from build123d import *

# Parameters (mm, degrees)
SKETCH1_R           = 4.5
BOSS_EXTRUDE1_DEPTH = 2.4
FILLET1_R           = 3
SKETCH2_R           = 3.25
BOSS_EXTRUDE2_DEPTH = 5.5


with BuildPart() as part:
    # Sketch1 → Boss-Extrude1 (new body)
    with BuildSketch(Plane(origin=(0, 0, 0), x_dir=(1, 0, 0), z_dir=(0, 1, 0))):
        with BuildLine():
            ThreePointArc((-48.371159118, 10.670216357), (-67.382417284, 0), (-48.371159118, -10.670216357))
            Line((-48.371159118, -10.670216357), (-39.699633202, -7.41775842))
            Line((-39.699633202, -7.41775842), (-5.857739229, -16.176946436))
            ThreePointArc((-5.857739229, -16.176946436), (21.617582716, 0), (-5.857739229, 16.176946436))
            Line((-5.857739229, 16.176946436), (-39.699633202, 7.41775842))
            Line((-39.699633202, 7.41775842), (-48.371159118, 10.670216357))
        make_face()
        with BuildLine():
            Line((-11.950545902, 3), (-25.528315318, 3))
            ThreePointArc((-25.528315318, 3), (-28.882417284, 4.5), (-32.23651925, 3))
            Line((-32.23651925, 3), (-42.747756184, 3))
            Line((-42.747756184, 3), (-17.634945081, 8.68439918))
            Line((-17.634945081, 8.68439918), (-11.950545902, 3))
        make_face(mode=Mode.SUBTRACT)
        with BuildLine():
            Line((9.717339795, -8.5), (9.717339795, 8.5))
            ThreePointArc((9.717339795, 8.5), (18.217339795, 0), (9.717339795, -8.5))
        make_face(mode=Mode.SUBTRACT)
        with BuildLine():
            Line((-42.747756184, -3), (-32.23651925, -3))
            ThreePointArc((-32.23651925, -3), (-28.882417284, -4.5), (-25.528315318, -3))
            Line((-25.528315318, -3), (-11.950545902, -3))
            Line((-11.950545902, -3), (-17.634945081, -8.68439918))
            Line((-17.634945081, -8.68439918), (-42.747756184, -3))
        make_face(mode=Mode.SUBTRACT)
        with Locations((-54.882417284, 0)):
            Circle(SKETCH1_R, mode=Mode.SUBTRACT)
    extrude(amount=BOSS_EXTRUDE1_DEPTH)

    # Fillet1
    fillet1_edges = [part.edges().sort_by_distance(p)[0] for p in [
        (-39.699633202, 1.2, -7.41775842),
        (-5.857739229, 1.2, -16.176946436),
        (-5.857739229, 1.2, 16.176946436),
        (-39.699633202, 1.2, 7.41775842),
    ]]
    fillet(fillet1_edges, radius=FILLET1_R)

    # Sketch2 → Boss-Extrude2 (add)
    with BuildSketch(Plane(origin=(0, 2.4, 0), x_dir=(1, 0, 0), z_dir=(0, 1, 0))):
        with Locations((-28.882417284, 0)):
            Circle(SKETCH2_R)
        with BuildLine():
            Line((-48.371159118, 8.621240559), (-48.371159118, 10.670216357))
            ThreePointArc((-48.371159118, 10.670216357), (-67.382417284, 0), (-48.371159118, -10.670216357))
            Line((-48.371159118, -10.670216357), (-48.371159118, -8.621240559))
            ThreePointArc((-48.371159118, -8.621240559), (-65.686225486, 0), (-48.371159118, 8.621240559))
        make_face()
        with BuildLine():
            Line((19.549259441, 8.5), (17.608614425, 8.5))
            ThreePointArc((17.608614425, 8.5), (19.917582716, 0), (17.608614425, -8.5))
            Line((17.608614425, -8.5), (19.549259441, -8.5))
            ThreePointArc((19.549259441, -8.5), (21.617582716, 0), (19.549259441, 8.5))
        make_face()
    extrude(amount=BOSS_EXTRUDE2_DEPTH)


solid = part.part
Source: CAD feature listing. Evaluate the final solid. Frame: model axes, mm. A direction names the side the tool comes from. Round coordinates to 2 decimals unless told otherwise and drop trailing zeros. Write each loop counter-clockwise with the first axis right and the second up, starting at its lowest first coordinate (ties: lowest second). Pieces come first, ordered by that corner, then holes. Notation, with made-up numbers: (88, 70) - (105, 70) arc R11 cw to (105, 84) - close; hole circle Ø1 at (13.25, -15). An arc over 180 degrees is marked (long way). Use CSV: the item, a comma, the result in double quotes. Start each with the question number.
(1) Material intervals for probe 1 along X at (y, z) = (5.75, -2); probe 2 along Z at (x, y) = (-41, 1); probe 3 along Z at (x, y) = (-17, 0.75), sorted ascending. Write a range as [from, to].
(2) First-contact query: pin 1 Ø1.2 at (x, y) = (-15.5, 1.5) entering from +Z; pin 2 Ø1 at (x, y) = (19, 4) entering from -Z; pin 3 Ø0.7 at (x, y) = (-39.5, 1) entering from +Z; pin 4 Ø2 at (x, z) = (-3.5, 7) entering from -Y. Flat tips, straight axial feed; report the tip coordinate or a pass-through.
(3) Cut plane C-C, the plane x = 12.5. Return loops of the section in (y, z).
(4) Cut plane A-A, the plane y = 6.5. Return loops of the section in (x, z), and give its area (3 significant figures).
(5) Cut plane B-B, the plane z = 0. Return loops of the section in (x, y), and give its area (3 significant figures).
(6) Mould query, pull axis Z, two halves, no side actions, for faces 4 (the face through (-44.42, 1.18, -9.19)), 5 (the face through (-29, 7.9, 0)), 6 (the face through (-65.68, 5.11, 0.34)), 7 (the face through (19.917, 5.111, -0.125)). Classes: pulls with the +Z half, pulls with the -Z half, needs draft (parallel to the pull), parting line crosses it, or undercut.
(7) Set-up query: faces 1 (the face through (-28.8, 1.2, -4.5)), 2 (the face through (-25.782, 5.111, -0.976)), 3 (the face through (19, 5, 8.5)). Return all of +Z, -Z, +X, -X, +Y, -Y with unobstructed straight access to the full face (end or side cutting, diameter ignored); none if empty.
Geometry says:
1,probe 1,"[-67.22, -65.5], [-31.44, -26.32], [19.8, 21.51]"
1,probe 2,"[-7.91, -3.4], [-3, 3], [3.4, 7.91]"
1,probe 3,"[-13.29, -8.05], [-3, 3], [8.05, 13.29]"
2,pin 1,"z = 13.84"
2,pin 2,"z = -8.5"
2,pin 3,"z = 7.58"
2,pin 4,"y = 0"
3,outline,"(0, -15.94) - (2.4, -15.94) - (2.4, -8.03) - (0, -8.03) - close; (0, 8.03) - (2.4, 8.03) - (2.4, 15.94) - (0, 15.94) - close"
4,outline,"(-48.37, -10.67) - (-48.37, -8.62) arc R10.8 cw (long way) to (-48.37, 8.62) - (-48.37, 10.67) arc R12.5 ccw (long way) to start; circle Ø6.5 at (-28.88, 0); (17.61, -8.5) - (19.55, -8.5) arc R18.5 ccw to (19.55, 8.5) - (17.61, 8.5) arc R16.8 cw to start"
4,area,"149 mm²"
5,outline,"(-67.38, 0) - (-59.38, 0) - (-59.38, 2.4) - (-65.69, 2.4) - (-65.69, 7.9) - (-67.38, 7.9) - close; (-50.38, 0) - (9.72, 0) - (9.72, 2.4) - (-25.63, 2.4) - (-25.63, 7.9) - (-32.13, 7.9) - (-32.13, 2.4) - (-50.38, 2.4) - close; (18.22, 0) - (21.62, 0) - (21.62, 7.9) - (19.92, 7.9) - (19.92, 2.4) - (18.22, 2.4) - close"
5,area,"226 mm²"
6,face 4,"pulls with the -Z half"
6,face 5,"needs draft"
6,face 6,"undercut"
6,face 7,"undercut"
7,face 1,"+Y, -Y"
7,face 2,"+Y"
7,face 3,"+Z, +X, +Y"
